Could you check a few things on this model? Use its own coordinates, in mm. Give positions to 0.01 mm unless a question says otherwise; leave off trailing zeros. Write each loop counter-clockwise with the first axis right and the second up, starting at its lowest first coordinate (ties: lowest second). Pieces come first, ordered by that corner, then holes. Notation, with made-up numbers: (68, 78) -> (109, 78) arc R16 cw to (109, 108) -> close; hole circle Ø1 at (-9, 85). An arc over 180 degrees is marked (long way). One line per question, with ' | ' between items.
Autodesk Inventor part; units mm, degrees
ref_plane "YZ Plane" through (0, 0, 0) normal (1, 0, 0) x (0, 1, 0)
ref_plane "XZ Plane" through (0, 0, 0) normal (0, 1, 0) x (-1, 0, 0)
ref_plane "XY Plane" through (0, 0, 0) normal (0, 0, 1) x (1, 0, 0)
sketch "Sketch1" plane through (0, 0, 0) normal (0, 0, 1) x (1, 0, 0)
  line L0 (0, 0) -> (146.5, 0)
  line L1 (146.5, 0) -> (146.5, 54)
  line L2 (146.5, 54) -> (0, 54)
  line L3 (0, 54) -> (0, 0)
  circle A0 centre (43.5, 16) radius 6
  circle A1 centre (65.5, 16) radius 6
  circle A2 centre (87.5, 16) radius 6
  circle A3 centre (109.5, 16) radius 6
  circle A4 centre (131.5, 16) radius 6
  circle A5 centre (43.5, 38) radius 6
  circle A6 centre (65.5, 38) radius 6
  circle A7 centre (87.5, 38) radius 6
  circle A8 centre (109.5, 38) radius 6
  circle A9 centre (131.5, 38) radius 6
  circle A10 centre (19.5, 27) radius 8
  line L4 (27, 19) -> (12, 19)
  line L5 (12, 19) -> (12, 35)
  line L6 (12, 35) -> (27, 35)
  line L7 (27, 35) -> (27, 19)
  line L8 (27, 19) -> (12, 35) construction
  line L9 (12, 19) -> (27, 35) construction
  point P0 (27, 24.2161)
  point P1 (12, 24.2161)
  point P2 (12, 29.7839)
  point P3 (27, 29.7839)
  dimension "d0" = 12
  dimension "d3" = 22
  dimension "d6" = 22
  dimension "d9" = 16
  dimension "d10" = 16
  dimension "d11" = 15
  dimension "d12" = 16
  dimension "d13" = 15
  dimension "d14" = 24
  dimension "d15" = 19.5
  dimension "d16" = 67
  dimension "d17" = 27
extrude "Extrusion1" add sketch "Sketch1" along normal blind 3 contours L3 L2 L1 L0 | A10 L7 | A10 L6 L7 | L7 L4 A10 | A10 L5 L6 | L4 L5 A10 | L5 A10
properties part number "button-front"
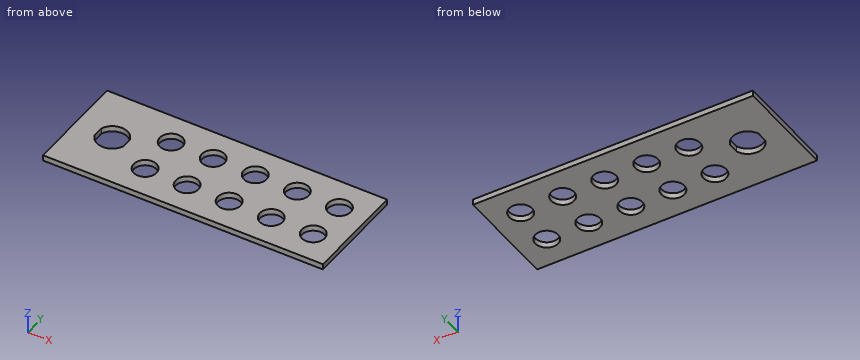
Q1. Will this pin go through, and if not, where does the flat tip stop? pin 1 (15.5 mm diameter, centred on x = 109.5, y = 38, fed in from -Z).
Answer below:
pin 1: stops at z = 0
Q2. Imagine slicing it at D-D on z = 2.2. Count the separate pieces of the cut face and the enclosed holes in it, and give its area (3 significant figures).
Answer below:
separate pieces: 1 | enclosed holes: 11 | area: 6,580 mm^2
Q3. Imagine slicing it at C-C on y = 27.5. Please give me the cut outline in (x, z).
Answer below:
outline: (0, 0) -> (12, 0) -> (12, 3) -> (0, 3) -> close; (27, 0) -> (146.5, 0) -> (146.5, 3) -> (27, 3) -> close
Q4. Imagine slicing it at B-B on x = 87.5. Please give me the cut outline in (y, z).
Answer below:
outline: (0, 0) -> (10, 0) -> (10, 3) -> (0, 3) -> close; (22, 0) -> (32, 0) -> (32, 3) -> (22, 3) -> close; (44, 0) -> (54, 0) -> (54, 3) -> (44, 3) -> close
Q5. If I drill on line 1 along Y through (x, z) = (109.5, 2.3); line 2 along Y through (x, z) = (61, 0.45); line 3 along X through (y, z) = (18, 1), over which ranges is the centre line in solid material (lowest first)?
Answer below:
line 1: y = 0 to 10, 22 to 32, 44 to 54 | line 2: y = 0 to 12.03, 19.97 to 34.03, 41.97 to 54 | line 3: x = 0 to 37.84, 49.16 to 59.84, 71.16 to 81.84, 93.16 to 103.84, 115.16 to 125.84, 137.16 to 146.5
Q6. Imagine slicing it at A-A on y = 38. Please give me the cut outline in (x, z), and give its area (4 significant figures).
Answer below:
outline: (0, 0) -> (37.5, 0) -> (37.5, 3) -> (0, 3) -> close; (49.5, 0) -> (59.5, 0) -> (59.5, 3) -> (49.5, 3) -> close; (71.5, 0) -> (81.5, 0) -> (81.5, 3) -> (71.5, 3) -> close; (93.5, 0) -> (103.5, 0) -> (103.5, 3) -> (93.5, 3) -> close; (115.5, 0) -> (125.5, 0) -> (125.5, 3) -> (115.5, 3) -> close; (137.5, 0) -> (146.5, 0) -> (146.5, 3) -> (137.5, 3) -> close | area: 259.5 mm^2
